from build123d import *

# Parameters (mm, degrees)
SKETCH2_W           = 85.09
SKETCH2_H           = 63.5
BOSS_EXTRUDE1_DEPTH = 1.27
SKETCH3_W           = 78.486
SKETCH3_H           = 56.896
BOSS_EXTRUDE2_DEPTH = 3.175
SKETCH4_W           = 50.8
SKETCH4_H           = 23.114
CUT_EXTRUDE1_DEPTH  = 1.778
SKETCH5_W           = 44.45
SKETCH5_H           = 23.114
CUT_EXTRUDE2_DEPTH  = 3.667
SKETCH6_R           = 1.4605
CUT_EXTRUDE3_DEPTH  = 5.445


with BuildPart() as part:
    # Sketch2 → Boss-Extrude1 (new body)
    with BuildSketch(Plane(origin=(0, 0, 0), x_dir=(1, 0, 0), z_dir=(0, 1, 0))):
        with Locations((42.545, 31.75)):
            Rectangle(SKETCH2_W, SKETCH2_H)
    extrude(amount=BOSS_EXTRUDE1_DEPTH)

    # Sketch3 → Boss-Extrude2 (add)
    with BuildSketch(Plane(origin=(0, 1.27, 0), x_dir=(1, 0, 0), z_dir=(0, 1, 0))):
        with Locations((42.545, 31.75)):
            Rectangle(SKETCH3_W, SKETCH3_H)
    extrude(amount=BOSS_EXTRUDE2_DEPTH)

    # Sketch4 → Cut-Extrude1 (cut)
    with BuildSketch(Plane(origin=(0, 4.445, 0), x_dir=(1, 0, 0), z_dir=(0, 1, 0))):
        with Locations((40.894, 31.75)):
            Rectangle(SKETCH4_W, SKETCH4_H)
    extrude(amount=-CUT_EXTRUDE1_DEPTH, mode=Mode.SUBTRACT)

    # Sketch5 → Cut-Extrude2 (cut, through all)
    with BuildSketch(Plane(origin=(0, 2.667, 0), x_dir=(1, 0, 0), z_dir=(0, 1, 0))):
        with Locations((40.894, 31.75)):
            Rectangle(SKETCH5_W, SKETCH5_H)
    extrude(amount=-CUT_EXTRUDE2_DEPTH, mode=Mode.SUBTRACT)

    # Sketch6 → Cut-Extrude3 (cut, through all)
    with BuildSketch(Plane(origin=(0, 4.445, 0), x_dir=(1, 0, 0), z_dir=(0, 1, 0))):
        with Locations((9.652, 53.848)):
            Circle(SKETCH6_R)
        with Locations((9.652, 9.652)):
            Circle(SKETCH6_R)
        with Locations((75.438, 53.848)):
            Circle(SKETCH6_R)
        with Locations((75.438, 9.652)):
            Circle(SKETCH6_R)
    extrude(amount=-CUT_EXTRUDE3_DEPTH, mode=Mode.SUBTRACT)


solid = part.part
CAD build for the part. Positions are in the model's coordinates, mm. A direction names the side the tool comes from. Give positions to 0.01 mm unless a question says otherwise; leave off trailing zeros. Order: outer loops, then holes, each group sorted by start corner. A loop starts at its lowest first (then second) coordinate and runs counter-clockwise, first axis right, second up. Notation, with made-up numbers: (7, -35.75) -> (58, -35.75) arc R4 cw to (58, -30.75) -> close; hole circle Ø6 at (-26, 27.25). An arc over 180 degrees is marked (long way). Return JSON: item names as keys, results as strings.
Q1. Mould opens along X. For faces 1 (the face through (42, 4.445, -20)), 2 (the face through (18.669, 1, -32)), 3 (the face through (3.302, 3, -31)) say: pulls with the +X half, pulls with the -X half, needs draft (parallel to the pull), parting line crosses it, or undercut.
Working result:
{"face 1": "needs draft", "face 2": "undercut", "face 3": "pulls with the -X half"}
Q2. Saw through at B-B (x = 35). Write the cut outline in (y, z) (3 decimals).
Working result:
{"outline": "(0, -63.5) -> (1.27, -63.5) -> (1.27, -60.198) -> (4.445, -60.198) -> (4.445, -43.307) -> (0, -43.307) -> close; (0, -20.193) -> (4.445, -20.193) -> (4.445, -3.302) -> (1.27, -3.302) -> (1.27, 0) -> (0, 0) -> close"}
Q3. Flat gauge pins, fed straight in: pin 1 (1.4 mm diameter, centred on y = 3.5, z = -28, fed in from -X); pin 2 (1 mm diameter, centred on x = 64, z = -33, fed in from +Y); pin 3 (0.5 mm diameter, centred on y = 4, z = -36.5, fed in from +X). Where does each tip first touch, or does it go through?
Working result:
{"pin 1": "x = 3.3", "pin 2": "y = 2.67", "pin 3": "x = 81.79"}
Q4. Which spindle directions (+Z, -Z, +X, -X, +Y, -Y) get a long thin tool onto all of the face, cutting with end or side? Do faces 4 (the face through (42, 3, -60.198)), 5 (the face through (42, 3, -3.302)), 6 (the face through (81.788, 3, -31)), 7 (the face through (17, 2.667, -32)). Say none if no direction does.
Working result:
{"face 4": "-Z, +X, -X, +Y", "face 5": "+Z, +X, -X, +Y", "face 6": "+Z, -Z, +X, +Y", "face 7": "+Y"}
Q5. Saw through at D-D (x = 12). Write the cut outline in (y, z) (3 decimals), then the cut area to 3 significant figures.
Working result:
{"outline": "(0, -63.5) -> (1.27, -63.5) -> (1.27, -60.198) -> (4.445, -60.198) -> (4.445, -3.302) -> (1.27, -3.302) -> (1.27, 0) -> (0, 0) -> close", "area": "261 mm²"}
Q6. Saw through at A-A (z = -29). Write the cut outline in (x, y) (3 decimals), then the cut area to 3 significant figures.
Working result:
{"outline": "(0, 0) -> (18.669, 0) -> (18.669, 2.667) -> (15.494, 2.667) -> (15.494, 4.445) -> (3.302, 4.445) -> (3.302, 1.27) -> (0, 1.27) -> close; (63.119, 0) -> (85.09, 0) -> (85.09, 1.27) -> (81.788, 1.27) -> (81.788, 4.445) -> (66.294, 4.445) -> (66.294, 2.667) -> (63.119, 2.667) -> close", "area": "148 mm²"}
Q7. Saw through at C-C (z = -45.5). Write the cut outline in (x, y) (3 decimals).
Working result:
{"outline": "(0, 0) -> (85.09, 0) -> (85.09, 1.27) -> (81.788, 1.27) -> (81.788, 4.445) -> (3.302, 4.445) -> (3.302, 1.27) -> (0, 1.27) -> close"}
Q8. Drill centre lines: line 1 (Z direction, x = 48, y = 2.6); line 2 (X direction, y = 2.35, z = -21); line 3 (X direction, y = 3.3, z = -42.5). Where is each one in solid material? Low to high.
Working result:
{"line 1": "-60.2 to -43.31, -20.19 to -3.3", "line 2": "3.3 to 18.67, 63.12 to 81.79", "line 3": "3.3 to 15.49, 66.29 to 81.79"}
